Design review of the part shown in the three views and the two pictorial views. Dimensions are in mm from the part's minimum x, y and z. A direction names the side the tool comes from. Give positions to 0.01 mm unless a question says otherwise; leave off trailing zeros. Write each loop counter-clockwise with the first axis right and the second up, starting at its lowest first coordinate (ties: lowest second). Pieces come first, ordered by that corner, then holes.
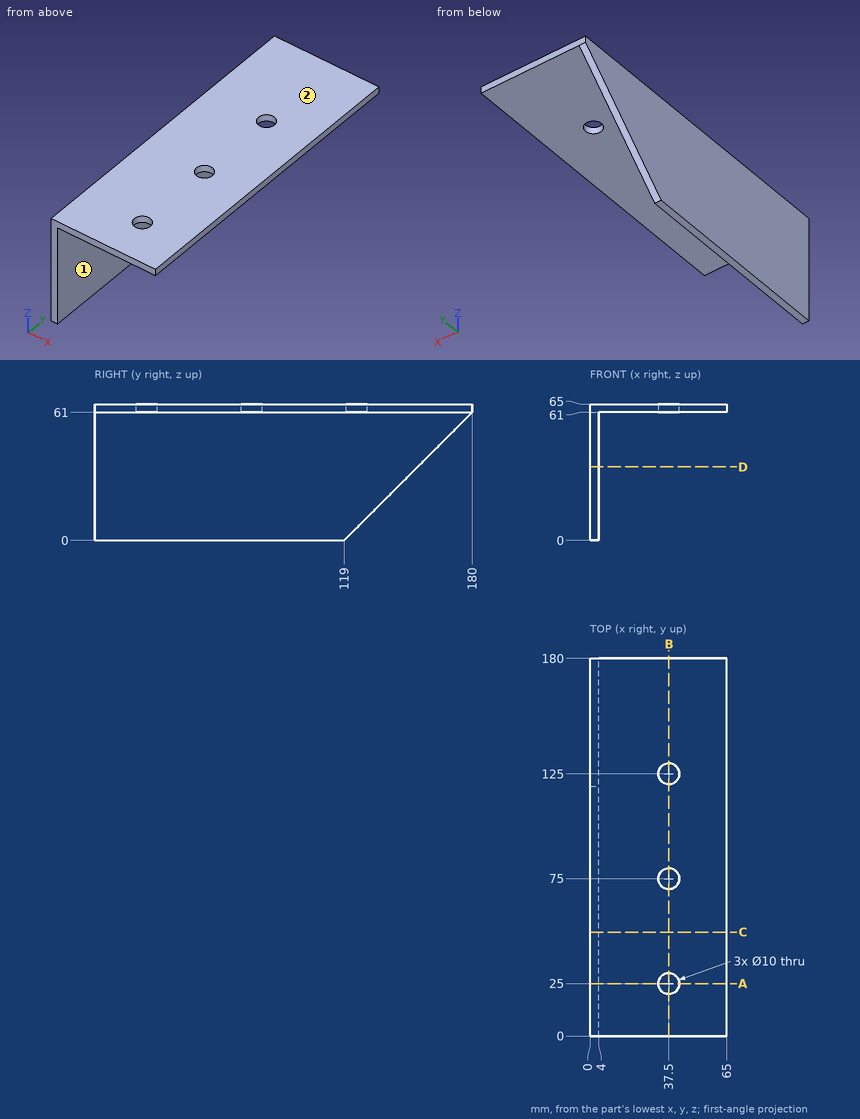
(1) Consider section C-C, the plane y = 49.5. Give the boundary of the cut face in (x, z).
Resolved:
outline: (0, 0) - (4, 0) - (4, 61) - (65, 61) - (65, 65) - (0, 65) - close
(2) Clearance check with flat-ended pins moving along their axes: P1, Ø5, axis at y = 27.5, z = 38, coming from the -X side; P2, Ø8, axis at x = 37.5, y = 125, coming from the -Z side; P3, Ø3, axis at x = 11.5, y = 40.5, coming from the -Z side; P4, Ø2, axis at y = 78.5, z = 25, coming from the +X side. State where each tip first meets the part, or that it passes through.
Resolved:
P1: stops at x = 0
P2: passes through
P3: stops at z = 61
P4: stops at x = 4
(3) Consider section B-B, the plane x = 37.5. Give the boundary of the cut face in (y, z).
Resolved:
outline: (0, 61) - (20, 61) - (20, 65) - (0, 65) - close; (30, 61) - (70, 61) - (70, 65) - (30, 65) - close; (80, 61) - (120, 61) - (120, 65) - (80, 65) - close; (130, 61) - (180, 61) - (180, 65) - (130, 65) - close
(4) Consider section D-D, the plane z = 35. Give the boundary of the cut face in (x, y), then the cut area to 3 significant figures.
Resolved:
outline: (0, 0) - (4, 0) - (4, 154) - (0, 154) - close
area: 616 mm2
(5) To check wall thickness, follow L1, parallel to Y at x = 37.5, z = 62.5; L2, parallel to X at y = 125, z = 63.5; L3, parallel to Z at x = 13, y = 67.5. State the ranges of each line that lie inside material, in increasing order.
Resolved:
L1: y = 0 to 20, 30 to 70, 80 to 120, 130 to 180
L2: x = 0 to 32.5, 42.5 to 65
L3: z = 61 to 65
(6) Consider section A-A, the plane y = 25. Give the boundary of the cut face in (x, z), then the cut area to 3 significant figures.
Resolved:
outline: (0, 0) - (4, 0) - (4, 61) - (32.5, 61) - (32.5, 65) - (0, 65) - close; (42.5, 61) - (65, 61) - (65, 65) - (42.5, 65) - close
area: 464 mm2
(7) Tool access review of the marked faces 1 and 2: name each direction out of +Z, -Z, +X, -X, +Y, -Y from which nothing blocks a thin tool from reaching the whole face with its end or side.
Resolved:
face 1: -Z, +X, +Y, -Y
face 2: +Z, +X, -X, +Y, -Y
